Autodesk Inventor part; units mm, degrees
ref_plane "YZ Plane" through (0, 0, 0) normal (1, 0, 0) x (0, 1, 0)
ref_plane "XZ Plane" through (0, 0, 0) normal (0, 1, 0) x (-1, 0, 0)
ref_plane "XY Plane" through (0, 0, 0) normal (0, 0, 1) x (1, 0, 0)
ref_plane "작업 평면1" through (0, 0, 0) normal (0, 0, 1) x (1, 0, 0)
sketch "스케치1" plane through (0, 0, 0) normal (0, 0, 1) x (1, 0, 0)
  arc A0 (20.1, 4.5766) -> (19.5808, 6.2636) centre (17.1, 4.5766) ccw
  line L0 (19.5808, 6.2636) -> (15.5953, 12.1246)
  arc A1 (15.5953, 12.1246) -> (13.9414, 13) centre (13.9414, 11) ccw
  line L1 (13, 13) -> (13.9414, 13)
  arc A2 (14.5, 11.5) -> (13, 13) centre (13, 11.5) ccw
  line L2 (14.5, -41.5) -> (14.5, 11.5)
  arc A3 (13.5, -42.5) -> (14.5, -41.5) centre (13.5, -41.5) ccw
  line L3 (-13.5, -42.5) -> (13.5, -42.5)
  arc A4 (-14.5, -41.5) -> (-13.5, -42.5) centre (-13.5, -41.5) ccw
  line L4 (-14.5, 11.5) -> (-14.5, -41.5)
  arc A5 (-13, 13) -> (-14.5, 11.5) centre (-13, 11.5) ccw
  line L5 (-13.9414, 13) -> (-13, 13)
  arc A6 (-13.9414, 13) -> (-15.5953, 12.1246) centre (-13.9414, 11) ccw
  line L6 (-15.5953, 12.1246) -> (-19.5808, 6.2636)
  arc A7 (-19.5808, 6.2636) -> (-20.1, 4.5766) centre (-17.1, 4.5766) ccw
  line L7 (-20.1, 4.5766) -> (-20.1, -39.6766)
  arc A8 (-20.1, -39.6766) -> (-19.5808, -41.3636) centre (-17.1, -39.6766) ccw
  line L8 (-19.5808, -41.3636) -> (-15.8929, -46.7869)
  arc A9 (-15.8929, -46.7869) -> (-13.4121, -48.1) centre (-13.4121, -45.1) ccw
  line L9 (-13.4121, -48.1) -> (13.4121, -48.1)
  arc A10 (13.4121, -48.1) -> (15.8929, -46.7869) centre (13.4121, -45.1) ccw
  line L10 (15.8929, -46.7869) -> (19.5808, -41.3636)
  arc A11 (19.5808, -41.3636) -> (20.1, -39.6766) centre (17.1, -39.6766) ccw
  line L11 (20.1, -39.6766) -> (20.1, 4.5766)
  circle A12 centre (-17.3, 4) radius 1.35
  circle A13 centre (-17.3, -18) radius 1.35
  circle A14 centre (-11, -45.3) radius 1.35
  circle A15 centre (17.3, 4) radius 1.35
  circle A16 centre (17.3, -18) radius 1.35
  circle A17 centre (11, -45.3) radius 1.35
  circle A18 centre (-17.3, -40) radius 1.35
  circle A19 centre (17.3, -40) radius 1.35
  arc A20 (14.6, 11.5) -> (12.2254, 12.9) centre (13, 11.5) ccw
  line L12 (12.2254, 12.9) -> (13.9414, 12.9)
  arc A21 (15.5126, 12.0684) -> (13.9414, 12.9) centre (13.9414, 11) ccw
  line L13 (15.5126, 12.0684) -> (15.8991, 11.5)
  line L14 (19.3671, -41.5) -> (15.8102, -46.7307)
  arc A22 (13.4121, -48) -> (15.8102, -46.7307) centre (13.4121, -45.1) ccw
  line L15 (13.4121, -48) -> (-13.4121, -48)
  arc A23 (-15.8102, -46.7307) -> (-13.4121, -48) centre (-13.4121, -45.1) ccw
  line L16 (-15.8102, -46.7307) -> (-19.4981, -41.3073)
  arc A24 (-20, -39.6766) -> (-19.4981, -41.3073) centre (-17.1, -39.6766) ccw
  line L17 (-20, -39.6766) -> (-20, 4.5766)
  arc A25 (-19.4981, 6.2073) -> (-20, 4.5766) centre (-17.1, 4.5766) ccw
  line L18 (-19.4981, 6.2073) -> (-15.5126, 12.0684)
  arc A26 (-13.9414, 12.9) -> (-15.5126, 12.0684) centre (-13.9414, 11) ccw
  line L19 (-13.9414, 12.9) -> (-12.2254, 12.9)
  arc A27 (-12.2254, 12.9) -> (-14.6, 11.5) centre (-13, 11.5) ccw
  line L20 (-14.6, 11.5) -> (-14.6, -41.5)
  arc A28 (-14.6, -41.5) -> (-13.5, -42.6) centre (-13.5, -41.5) ccw
  line L21 (-13.5, -42.6) -> (13.5, -42.6)
  arc A29 (13.5, -42.6) -> (14.6, -41.5) centre (13.5, -41.5) ccw
  line L22 (14.6, -41.5) -> (14.6, 11.5)
  line L23 (14.6, 11.5) -> (39.6, 11.5)
  line L24 (39.6, -41.5) -> (14.6, -41.5)
  line L25 (14.6, -41.5) -> (14.6, 11.5)
  circle A30 centre (17.3, 4) radius 1.35
  circle A31 centre (17.3, -18) radius 1.35
  line L26 (45.5, -39.6766) -> (45.5, -37.525)
  line L27 (47.5, -37.525) -> (45.5, -37.525)
  line L28 (47.5, -36.025) -> (47.5, -37.525)
  line L29 (47.5, -36.025) -> (45, -36.025)
  line L30 (45, -36.025) -> (45, -21.975)
  line L31 (47.5, -21.975) -> (45, -21.975)
  line L32 (47.5, -21.975) -> (47.5, -20.475)
  line L33 (47.5, -20.475) -> (45.5, -20.475)
  line L34 (45.5, -20.475) -> (45.5, -15.525)
  line L35 (47.5, -15.525) -> (45.5, -15.525)
  line L36 (47.5, -15.525) -> (47.5, -14.025)
  line L37 (47.5, -14.025) -> (45, -14.025)
  line L38 (45, -14.025) -> (45, 0.025)
  line L39 (47.5, 0.025) -> (45, 0.025)
  line L40 (47.5, 0.025) -> (47.5, 1.525)
  line L41 (47.5, 1.525) -> (45.5, 1.525)
  line L42 (45.5, 1.525) -> (45.5, 4.5766)
  line L43 (43, 4.5766) -> (45.5, 4.5766)
  line L44 (43, -39.6766) -> (43, 4.5766)
  line L45 (43, -39.6766) -> (45.5, -39.6766)
  line L46 (14.6, 11.5) -> (43, 11.5)
  line L47 (43, 11.5) -> (43, -41.5)
  line L48 (43, -41.5) -> (14.6, -41.5)
  line L49 (14.6, -41.5) -> (14.6, 11.5)
  line L50 (45.5, -19.35) -> (45.5, -16.65)
  line L51 (43, -19.35) -> (43, -16.65)
  line L52 (43, -19.35) -> (43, -16.65)
  line L53 (43, -19.35) -> (43, -16.65)
  line L54 (47.5, -18) -> (45.5, -18)
  line L55 (47.5, 4) -> (45.5, 4)
  line L56 (33.5, 1) -> (36.5, 7) construction
  line L57 (36.5, 1) -> (33.5, 7) construction
  line L58 (33.9, 1.4) -> (36.1, 6.6) construction
  point P0 (0, 0)
  point P1 (19.488, -41.5)
  point P2 (16.02, 11.5)
  dimension "d0" = 0.1
  dimension "d1" = 25
  dimension "d2" = 53
  dimension "d3" = 2.7
  dimension "d4" = 2.7
  dimension "d5" = 3
  dimension "d6" = 6
extrude "돌출4" add sketch "스케치1" along normal blind 6 contours L11 A11 L10 L24 L22 L23 L0 A0 | A0 L0 L23 L46 L47 L44 L48 L24 L10 A11 L11 | A19
sketch "스케치3" plane through (43, -41.5, 0) normal (1, 0, 0) x (0, 0, -1)
  arc A0 (-5.0808, 47.7636) -> (-5.6, 46.0766) centre (-2.6, 46.0766) ccw
  line L0 (-5.6, 1.8234) -> (-5.6, 46.0766)
  arc A1 (-5.6, 1.8234) -> (-5.0808, 0.1364) centre (-2.6, 1.8234) ccw
  line L1 (-1.3929, -5.2869) -> (-5.0808, 0.1364)
  arc A2 (-1.3929, -5.2869) -> (1.0879, -6.6) centre (1.0879, -3.6) ccw
  line L2 (27.9121, -6.6) -> (1.0879, -6.6)
  arc A3 (27.9121, -6.6) -> (30.3929, -5.2869) centre (27.9121, -3.6) ccw
  line L3 (34.0808, 0.1364) -> (30.3929, -5.2869)
  arc A4 (34.0808, 0.1364) -> (34.6, 1.8234) centre (31.6, 1.8234) ccw
  line L4 (34.6, 46.0766) -> (34.6, 1.8234)
  arc A5 (34.6, 46.0766) -> (34.0808, 47.7636) centre (31.6, 46.0766) ccw
  line L5 (30.0953, 53.6246) -> (34.0808, 47.7636)
  arc A6 (30.0953, 53.6246) -> (28.4414, 54.5) centre (28.4414, 52.5) ccw
  line L6 (22.15, 54.5) -> (28.4414, 54.5)
  arc A7 (23.65, 53) -> (22.15, 54.5) centre (22.15, 53) ccw
  line L7 (23.65, 53) -> (23.65, 51.5)
  arc A8 (23.65, 51.5) -> (26, 49.15) centre (26, 51.5) ccw
  line L8 (26, 49.15) -> (28, 49.15)
  arc A9 (29, 48.15) -> (28, 49.15) centre (28, 48.15) ccw
  line L9 (29, 48.15) -> (29, 5.35)
  arc A10 (28, 4.35) -> (29, 5.35) centre (28, 5.35) ccw
  line L10 (28, 4.35) -> (26, 4.35)
  arc A11 (26, 4.35) -> (23.65, 2) centre (26, 2) ccw
  line L11 (23.65, 2) -> (23.65, 0)
  arc A12 (22.65, -1) -> (23.65, 0) centre (22.65, 0) ccw
  line L12 (22.65, -1) -> (6.35, -1)
  arc A13 (5.35, 0) -> (6.35, -1) centre (6.35, 0) ccw
  line L13 (5.35, 0) -> (5.35, 2)
  arc A14 (5.35, 2) -> (3, 4.35) centre (3, 2) ccw
  line L14 (3, 4.35) -> (1, 4.35)
  arc A15 (0, 5.35) -> (1, 4.35) centre (1, 5.35) ccw
  line L15 (0, 5.35) -> (0, 48.15)
  arc A16 (1, 49.15) -> (0, 48.15) centre (1, 48.15) ccw
  line L16 (1, 49.15) -> (3, 49.15)
  arc A17 (3, 49.15) -> (5.35, 51.5) centre (3, 51.5) ccw
  line L17 (5.35, 51.5) -> (5.35, 53)
  arc A18 (6.85, 54.5) -> (5.35, 53) centre (6.85, 53) ccw
  line L18 (0.5586, 54.5) -> (6.85, 54.5)
  arc A19 (0.5586, 54.5) -> (-1.0953, 53.6246) centre (0.5586, 52.5) ccw
  line L19 (-5.0808, 47.7636) -> (-1.0953, 53.6246)
  circle A20 centre (31.8, 45.5) radius 1.35
  circle A21 centre (31.8, 23.5) radius 1.35
  circle A22 centre (25.5, -3.8) radius 1.35
  circle A23 centre (-2.8, 45.5) radius 1.35
  circle A24 centre (-2.8, 23.5) radius 1.35
  circle A25 centre (3.5, -3.8) radius 1.35
  circle A26 centre (31.8, 1.5) radius 1.35
  circle A27 centre (-2.8, 1.5) radius 1.35
  circle A28 centre (-2.8, 45.5) radius 1.35
  circle A29 centre (-2.8, 23.5) radius 1.35
  point P0 (0, 41.5)
extrude "돌출5" cut sketch "스케치3" against normal blind 15 contours A23 | A24
sketch "스케치4" plane through (0, 0, 6) normal (0, 0, 1) x (1, 0, 0)
  line L0 (36.1, 1.4) -> (33.9, 1.4)
  line L1 (33.9, 1.4) -> (33.9, 6.6)
  line L2 (33.9, 6.6) -> (36.1, 6.6)
  line L3 (36.1, 6.6) -> (36.1, 1.4)
  line L4 (36.1, 1.4) -> (33.9, 6.6) construction
  line L5 (33.9, 1.4) -> (36.1, 6.6) construction
  line L6 (43, -16.65) -> (28, -16.65)
  line L7 (43, -19.35) -> (28, -19.35)
  line L8 (33.9, -20.6) -> (36.1, -20.6)
  line L9 (36.1, -20.6) -> (36.1, -15.4)
  line L10 (36.1, -15.4) -> (33.9, -15.4)
  line L11 (33.9, -15.4) -> (33.9, -20.6)
  line L12 (33.9, -20.6) -> (36.1, -15.4) construction
  line L13 (36.1, -20.6) -> (33.9, -15.4) construction
  point P0 (0, 0)
  point P1 (35, 4)
  point P2 (35, -18)
  dimension "d22" = 2.2
  dimension "d23" = 5.2
  dimension "d24" = 2.2
  dimension "d25" = 5.2
extrude "돌출6" cut sketch "스케치4" against normal blind 6
sketch "스케치5" plane through (0, 0, 6) normal (0, 0, 1) x (1, 0, 0)
  line L0 (33.9, 1.4) -> (33.9, 6.6)
  line L1 (33.9, 6.6) -> (36.1, 6.6)
  line L2 (36.1, 6.6) -> (36.1, 1.4)
  line L3 (36.1, 1.4) -> (33.9, 1.4)
  line L4 (36.1, -20.6) -> (33.9, -20.6)
  line L5 (33.9, -20.6) -> (33.9, -15.4)
  line L6 (33.9, -15.4) -> (36.1, -15.4)
  line L7 (36.1, -15.4) -> (36.1, -20.6)
  line L8 (14.6, -41.5) -> (43, -41.5)
  line L9 (43, -41.5) -> (43, 11.5)
  line L10 (43, 11.5) -> (14.6, 11.5)
  line L11 (14.6, 11.5) -> (14.6, -41.5)
  circle A0 centre (17.3, 4) radius 1.35
  circle A1 centre (17.3, -18) radius 1.35
  line L12 (43, -41.5) -> (14.6, -41.5)
  line L13 (14.6, -41.5) -> (14.6, -34.5)
  line L14 (14.6, -34.5) -> (43, -34.5)
  line L15 (43, -34.5) -> (43, -41.5)
  point P0 (0, 0)
  dimension "d28" = 7
extrude "돌출7" cut sketch "스케치5" against normal blind 10 contours L11 L14 L9 L8
sketch "스케치7" plane through (0, 0, 6) normal (0, 0, 1) x (1, 0, 0)
  circle A0 centre (17.3, -40) radius 1.35
  circle A1 centre (11, -45.3) radius 1.35
  circle A2 centre (-11, -45.3) radius 1.35
  circle A3 centre (-17.3, -40) radius 1.35
  line L0 (-13.4121, -48.1) -> (13.4121, -48.1)
  line L1 (-13, -42.5) -> (13, -42.5)
  line L2 (20.1, -39.6766) -> (20.1, 4.5766)
  line L3 (14.5, -41) -> (14.5, 11)
  line L4 (14.6, 11.5) -> (14.6, -34.5)
  line L5 (14.6, -34.5) -> (43, -34.5)
  line L6 (20, -39.6766) -> (20, 4.5766)
  line L7 (14.6, -41) -> (14.6, 11)
  line L8 (-13, -42.6) -> (13, -42.6)
  line L9 (-13.4121, -48) -> (13.4121, -48)
  line L10 (14.6, -34.5) -> (20, -34.5)
  line L11 (20, -34.5) -> (20, -42.6)
  line L12 (14.6, -42.6) -> (14.6, -34.5)
  line L13 (14.6, -42.6) -> (0, -42.6)
  line L14 (0, -42.6) -> (0, -48)
  line L15 (0, -48) -> (14.6, -48)
  line L16 (20, -42.6) -> (14.6, -48)
  circle A4 centre (17.3, -40) radius 1.35
  circle A5 centre (11, -45.3) radius 1.35
  point P0 (0, 0)
  point P1 (41, -34.5)
  point P2 (20, -34.5)
  point P3 (13, -42.6)
  point P4 (0, -42.6)
  point P5 (13.4121, -48)
  dimension "d33" = 0.1
  dimension "d35" = 0.1
  dimension "d36" = 0.1
  dimension "d37" = 0.1
extrude "돌출8" add sketch "스케치7" against normal blind 6 contours L5 L6 L11 L16 L15 L9 L14 L8 L13 L12 L7
fillet "모깎기5" radius 1 1 edges at (14.6, -42.6, 3)
sketch "스케치8" plane through (0, 0, 6) normal (0, 0, 1) x (1, 0, 0)
  circle A0 centre (11, -45.3) radius 1.35
  circle A1 centre (17.3, -40) radius 1.35
  circle A2 centre (17.3, -18) radius 1.35
  circle A3 centre (17.3, 4) radius 1.35
  line L0 (36.1, -20.6) -> (33.9, -20.6)
  line L1 (33.9, -20.6) -> (33.9, -15.4)
  line L2 (33.9, -15.4) -> (36.1, -15.4)
  line L3 (36.1, -15.4) -> (36.1, -20.6)
  line L4 (33.9, 1.4) -> (33.9, 6.6)
  line L5 (33.9, 6.6) -> (36.1, 6.6)
  line L6 (36.1, 6.6) -> (36.1, 1.4)
  line L7 (36.1, 1.4) -> (33.9, 1.4)
  line L8 (14.6, -48) -> (20, -42.6)
  line L9 (20, -42.6) -> (20, -34.5)
  line L10 (20, -34.5) -> (43, -34.5)
  line L11 (43, -34.5) -> (43, 11.5)
  line L12 (43, 11.5) -> (14.6, 11.5)
  line L13 (14.6, 11.5) -> (14.6, -41.6)
  arc A4 (13.6, -42.6) -> (14.6, -41.6) centre (13.6, -41.6) ccw
  line L14 (13.6, -42.6) -> (0, -42.6)
  line L15 (0, -48) -> (14.6, -48)
  line L16 (0, -42.6) -> (0, -48)
  line L17 (43, -34.5) -> (19.4142, -34.5)
  line L18 (19.4142, -34.5) -> (19.4142, -43.1858)
  line L19 (14.6, -48) -> (43, -34.5)
  line L20 (19.4142, -43.1858) -> (14.6, -48)
  point P0 (0, 0)
extrude "돌출12" add sketch "스케치8" against normal blind 6 contours L8 L9 L10 L19
mirror "미러2" about plane through (0, -48, 6) normal (-1, 0, 0)
properties part number "connecting plate under body" material "PMMA 플라스틱"
The model under review builds one solid part; all positions refer to its coordinate system, in mm. A direction names the side the tool comes from. Coordinates: 2 decimals unless noted, no trailing zeros. Write each loop counter-clockwise with the first axis right and the second up, starting at its lowest first coordinate (ties: lowest second). Pieces come first, ordered by that corner, then holes. Notation, with made-up numbers: (84.25, 0) -> (118.25, 0) arc R20 ccw to (118.25, 4) -> close; hole circle Ø8 at (-38, 11). An arc over 180 degrees is marked (long way). One line per item, written item: value. Start each with the question number.
Q1. The part is to be moulded in two halves that separate along Z. For faces 1 (the face through (-39.6, 5.2, 2.18)), 2 (the face through (39.6, 2.8, 2.18)), 3 (the face through (-36.1, 4, 4.4)), 4 (the face through (-20, -18, 6)), say which applies: +Z half, -Z half, draft (parallel to the pull), parting line (faces both ways), or undercut.
Q2. Add section C-C, the plane x = -32.5. Give the boundary of the cut face in (y, z).
Q3. To check wall thickness, follow probe 1 along X at (y, z) = (-16.5, 4.4); probe 2 along Y at (x, z) = (-11, 3.05); probe 3 along X at (y, z) = (-12, 2.95). State the ranges of each line that lie inside material, in increasing order.
Q4. For faces 5 (the face through (-14.6, -15, 3)), 6 (the face through (36.1, 4, 4.4)), 7 (the face through (-28, 4, 3)), 8 (the face through (39.598, -17.594, 1.512)), list the 3-axis set-ups (+Z, -Z, +X, -X, +Y, -Y) from which the entire face can be reached by the end or side of a thin tool; tool diameter is ignored.
Q5. Add section D-D, the plane z = 2.8. Count the separate pieces of the cut face and the enclosed holes in it, then the cut area to 3 significant figures.
Q6. Add section B-B, the plane x = 17.3. Give the boundary of the cut face in (y, z), then the cut area to 3 significant figures.
Q7. Add section A-A, the plane y = -26. Give the boundary of the cut face in (x, z), then the cut area to 3 significant figures.
Q8. Clearance check with flat-ended pins moving along their axes: P1, Ø3, axis at x = -5, z = 4, coming from the +Y side; P2, Ø1.6, axis at y = -18, z = 2.8, coming from the +X side; P3, Ø2, axis at x = -17.3, y = -18, coming from the -Z side; P4, Ø2.5, axis at y = 4, z = 2.8, coming from the -X side. State where each tip first meets the part, or that it passes through.
Response:
1. face 1: undercut
1. face 2: undercut
1. face 3: draft
1. face 4: +Z half
2. outline: (-39.49, 0) -> (11.5, 0) -> (11.5, 6) -> (-39.49, 6) -> close; hole circle Ø2.7 at (-18, 2.8); hole circle Ø2.7 at (4, 2.8)
3. probe 1: -43 to -36.1, -33.9 to -14.6, 14.6 to 33.9, 36.1 to 43
3. probe 2: -48 to -46.65, -43.95 to -42.6
3. probe 3: -43 to -14.6, 14.6 to 43
4. face 5: +Z, -Z, +Y
4. face 6: +Z, -Z
4. face 7: -X
4. face 8: +X
5. separate pieces: 1
5. enclosed holes: 8
5. area: 2,920 mm²
6. outline: (-46.72, 0) -> (-41.35, 0) -> (-41.35, 6) -> (-46.72, 6) -> close; (-38.65, 0) -> (-19.35, 0) -> (-19.35, 6) -> (-38.65, 6) -> close; (-16.65, 0) -> (2.65, 0) -> (2.65, 6) -> (-16.65, 6) -> close; (5.35, 0) -> (11.5, 0) -> (11.5, 6) -> (5.35, 6) -> close
6. area: 301 mm²
7. outline: (-43, 0) -> (-14.6, 0) -> (-14.6, 6) -> (-43, 6) -> close; (14.6, 0) -> (43, 0) -> (43, 6) -> (14.6, 6) -> close
7. area: 341 mm²
8. P1: y = -42.6
8. P2: x = 28
8. P3: through
8. P4: x = -28
